```python
from build123d import *

# Parameters (mm, degrees)
F0_W     = 48.063562
F0_H     = 3.309766
F1_DEPTH = 15.5
F2_R     = 2.565149
F2_R_2   = 2.584627
F2_R_3   = 2.54946
F2_R_4   = 2.565151
F2_R_5   = 2.47358
F2_R_6   = 2.509808
F2_R_7   = 2.553392
F2_R_8   = 2.553391
F3_DEPTH = 3
F4_W     = 16.371909
F4_H     = 15.5
F4_W_2   = 15.93889
F5_DEPTH = 0.1
F6_W     = 16.152791
F6_H     = 15.5
F6_W_2   = 8.003426
F7_DEPTH = 0.5
F8_W     = 8.105978
F8_H     = 15.5
F9_DEPTH = 0.4


with BuildPart() as f1:
    # F0 (on Front) → F1 (new body)
    with BuildSketch(Plane.XZ):
        with Locations((-1.726834, 1.654883)):
            Rectangle(F0_W, F0_H)
    extrude(amount=F1_DEPTH)

    # F2 (on face) → F3 (join)
    with BuildSketch(Plane.XY.offset(3.309766)):
        with Locations((-21.72962, -4.037504)):
            Circle(F2_R)
        with Locations((-21.72962, -11.402613)):
            Circle(F2_R_2)
        with Locations((-13.656328, -11.402613)):
            Circle(F2_R_3)
        with Locations((-13.656328, -4.037504)):
            Circle(F2_R)
        with Locations((-5.441401, -4.037504)):
            Circle(F2_R_4)
        with Locations((-5.441401, -11.402613)):
            Circle(F2_R_5)
        with Locations((1.923707, -11.402613)):
            Circle(F2_R_6)
        with Locations((1.923707, -4.037504)):
            Circle(F2_R_3)
        with Locations((9.997, -4.037504)):
            Circle(F2_R_3)
        with Locations((9.997, -11.402613)):
            Circle(F2_R_7)
        with Locations((18.211929, -11.402613)):
            Circle(F2_R_2)
        with Locations((18.211929, -4.037504)):
            Circle(F2_R_8)
    extrude(amount=F3_DEPTH)

    # F4 (on face) → F5 (join)
    with BuildSketch(Plane(origin=(0, 0, 0), x_dir=(1, 0, 0), z_dir=(0, 0, -1))):
        with Locations((14.118992, 7.75)):
            Rectangle(F4_W, F4_H)
        with Locations((-17.78917, 7.75)):
            Rectangle(F4_W_2, F4_H)
    extrude(amount=F5_DEPTH)

    # F6 (on face) → F7 (join)
    with BuildSketch(Plane.XY.offset(3.309766)):
        with Locations((-17.682219, -7.75)):
            Rectangle(F6_W, F6_H)
        with Locations((18.303234, -7.75)):
            Rectangle(F6_W_2, F6_H)
    extrude(amount=F7_DEPTH)

    # F8 (on face) → F9 (join)
    with BuildSketch(Plane.XY.offset(3.309766)):
        with Locations((-5.552835, -7.75)):
            Rectangle(F8_W, F8_H)
    extrude(amount=F9_DEPTH)


solid = f1.part
```
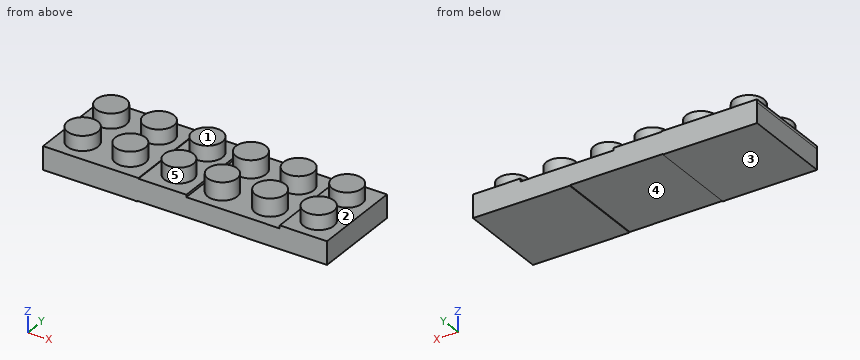
Here's how the part is built. I have some questions about the finished solid (model axes, mm). Face numbers are marked on the shaded views. A direction names the side the tool comes from. Round coordinates to 2 decimals unless told otherwise and drop trailing zeros. Order: outer loops, then holes, each group sorted by start corner. A loop starts at its lowest first (then second) coordinate and runs counter-clockwise, first axis right, second up. Notation, with made-up numbers: (63, 10.5) -> (76, 10.5) arc R19 ccw to (76, 38.5) -> close; hole circle Ø7 at (-12.5, 80). An arc over 180 degrees is marked (long way). Use a Markdown table: item, result. Add a question column.
(1) Suppose I cut it at D-D, the plane x = 18.5. Please give me the cut outline in (y, z), and give its area (3 significant figures).
(2) Suppose I cut it at C-C, the plane x = 10.5. Please give me the cut outline in (y, z), and give its area (3 significant figures).
(3) Suppose I cut it at A-A, the plane z = 4.5. Count the separate pieces of the cut face and the enclosed holes in it, and give its area (3 significant figures).
(4) If we mould it in two halves opening along X, with no side actions, what happens to the marked faces 1 and 2? For each: released by +X, released by -X, zero draft, split by the parting line, or undercut.
(5) I need wall thicknesses on line 1 along X through (y, z) = (-12.75, 3.5); line 2 along X through (y, z) = (-9.75, 3.5); line 3 along X through (y, z) = (-11.75, 4.25). Which ranges of each line are inside material? Lowest first, please.
(6) Suppose I cut it at B-B, the plane y = -0.75. Please give me the cut outline in (x, z), and give its area (3 significant figures).
(7) For pin 1 Ø4 at (x, y) = (1, -8.5) entering from -Z, with a flat end and sliding along its axis, tell me the tip position at first contact or that it passes through.
(8) For the marked faces 3, 4 and 5, which set-ups out of +Z, -Z, +X, -X, +Y, -Y let a thin tool reach every point of the face, with its end or its side?
Verdict:
| question | item | result |
|---|---|---|
| 1 | outline | (-15.5, -0.1) -> (0, -0.1) -> (0, 3.81) -> (-1.5, 3.81) -> (-1.5, 6.31) -> (-6.57, 6.31) -> (-6.57, 3.81) -> (-8.83, 3.81) -> (-8.83, 6.31) -> (-13.97, 6.31) -> (-13.97, 3.81) -> (-15.5, 3.81) -> close |
| 1 | area | 86.1 mm2 |
| 2 | outline | (-15.5, -0.1) -> (0, -0.1) -> (0, 3.31) -> (-1.54, 3.31) -> (-1.54, 6.31) -> (-6.54, 6.31) -> (-6.54, 3.31) -> (-8.9, 3.31) -> (-8.9, 6.31) -> (-13.91, 6.31) -> (-13.91, 3.31) -> (-15.5, 3.31) -> close |
| 2 | area | 82.9 mm2 |
| 3 | separate pieces | 12 |
| 3 | enclosed holes | 0 |
| 3 | area | 245 mm2 |
| 4 | face 1 | zero draft |
| 4 | face 2 | undercut |
| 5 | line 1 | -25.76 to -1.5, -0.19 to 4.04, 7.83 to 12.17, 14.3 to 22.3 |
| 5 | line 2 | -25.76 to -1.5, 0.03 to 3.81, 8.05 to 11.94, 14.3 to 22.3 |
| 5 | line 3 | -24.29 to -19.17, -16.18 to -11.13, -7.89 to -2.99, -0.56 to 4.41, 7.47 to 12.53, 15.65 to 20.77 |
| 6 | outline | (-25.76, -0.1) -> (-9.82, -0.1) -> (-9.82, 0) -> (5.93, 0) -> (5.93, -0.1) -> (22.3, -0.1) -> (22.3, 3.81) -> (14.3, 3.81) -> (14.3, 3.31) -> (-1.5, 3.31) -> (-1.5, 3.71) -> (-9.61, 3.71) -> (-9.61, 3.81) -> (-25.76, 3.81) -> close |
| 6 | area | 178 mm2 |
| 7 | pin 1 | z = 0 |
| 8 | face 3 | -Z, +X, -X, +Y, -Y |
| 8 | face 4 | -Z, +Y, -Y |
| 8 | face 5 | +Z |
